from build123d import *

# Parameters (mm, degrees)
PAD_DEPTH = 2.3


with BuildPart() as pad:
    # Sketch001 → Pad (new body, symmetric)
    with BuildSketch(Plane.YZ):
        with BuildLine():
            Line((5, 0), (5, 12))
            Line((5, 12), (8.5, 12))
            Line((8.5, 12), (12.715243, 19.841011))
            ThreePointArc((22.081098, 12.601746), (21.669324, 21.747216), (12.715243, 19.841011))
            Line((8.5, 0), (22.081098, 12.601746))
            Line((5, 0), (8.5, 0))
        make_face()
        with BuildLine():
            Line((-22.081101, 12.60177), (-8.500026, 0))
            Line((-8.500026, 0), (-5.000026, 0))
            Line((-5.000026, 0), (-5.000026, 12))
            Line((-5.000026, 12), (-8.500026, 12))
            Line((-8.500026, 12), (-12.71524, 19.841026))
            ThreePointArc((-12.71524, 19.841026), (-21.66932, 21.747241), (-22.081101, 12.60177))
        make_face()
    extrude(amount=PAD_DEPTH, both=True)


with BuildPart() as obj1:
    # Sketch → Revolution (revolve)
    with BuildSketch(Plane.YZ):
        Polygon((5, 0), (4.19, 0.467654), (4.19, 11.532346), (5, 12), (7.5, 12), (8.5, 0), align=None)
    revolve(axis=Axis((0, 0, 0), (0, 0, 1)))

    # Fusion: union Pad
    add(pad.part)


solid = obj1.part
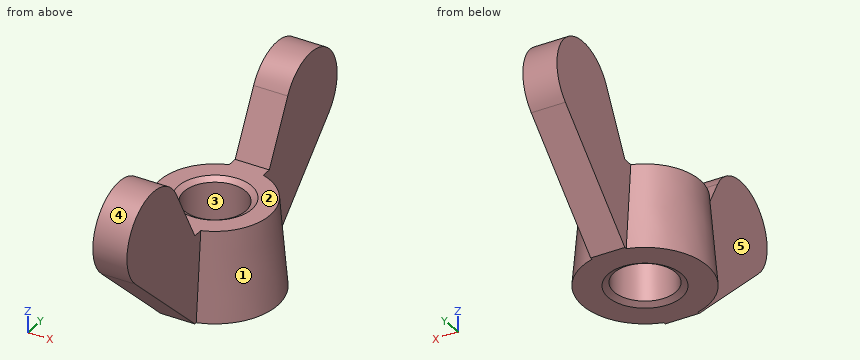
Input: part model. Units: mm. Frame: model coordinates. Face numbers are marked on the shaded views. A direction names the side the tool comes from. Coordinates: 2 decimals unless noted, no trailing zeros. Loops run counter-clockwise (first coordinate to the right, second up) from the corner with the lowest first, then second, coordinate; pieces in that order, holes last. Notation, with made-up numbers: (-8.5, 3.25) - (46.5, 3.25) arc R28 ccw to (46.5, 35.25) - close; hole circle Ø1 at (17, -17.5). An arc over 180 degrees is marked (long way). Answer in a Markdown table with one row per item. Add a question column.
Item 1: Access query for the marked faces 1 and 2. Directions: +Z, -Z, +X, -X, +Y, -Y. A direction counts if a zero-diameter tool reaches every point of the face in a straight line with its end or side. Return the directions, or none.
Item 2: Contact query for flat-ended pins moving along their axis: P1, Ø5, axis at y = -15, z = 10.5, coming from the -X side; P2, Ø5, axis at y = 14.5, z = 15, coming from the +X side; P3, Ø9.5, axis at x = 0, y = 0, coming from the -Z side. Output: stop coordinate, or through.
Item 3: Section query B-B on z = 17.25. Return the cut outline in (x, y).
Item 4: Section query A-A on x = 0. Return the cut outline in (y, z), then the cut area to 3 significant figures.
Item 5: Section query D-D on y = 16. Return the cut outline in (x, z).
Item 6: Section query C-C on z = 10.5. Return the cut outline in (x, y) (3 decimals).
Item 7: Mould query, pull axis X, two halves, no side actions, for the marked faces 3, 4 and 5. Classes: released by +X, released by -X, zero draft, split by the parting line, or undercut.
Item 8: Line query: line 1 along Y through (x, z) = (0, 3.75); line 2 along X through (y, z) = (1, 3); line 3 along X through (y, z) = (11.5, 17.25). Output: solid intervals per line, ascending. Write a range as [from, to].
Recorded:
| question | item | result |
|---|---|---|
| 1 | face 1 | +Z, +X |
| 1 | face 2 | +Z, +X, -X |
| 2 | P1 | x = -2.3 |
| 2 | P2 | x = 2.3 |
| 2 | P3 | z = 0.14 |
| 3 | outline | (-2.3, -23.99) - (2.3, -23.99) - (2.3, -11.32) - (-2.3, -11.32) - close; (-2.3, 11.32) - (2.3, 11.32) - (2.3, 23.99) - (-2.3, 23.99) - close |
| 4 | outline | (-22.08, 12.6) - (-8.5, 0) - (-5, 0) - (-4.19, 0.47) - (-4.19, 11.53) - (-5, 12) - (-8.5, 12) - (-12.72, 19.84) arc R6 ccw (long way) to start; (4.19, 0.47) - (5, 0) - (8.5, 0) - (22.08, 12.6) arc R6 ccw (long way) to (12.72, 19.84) - (8.5, 12) - (5, 12) - (4.19, 11.53) - close |
| 4 | area | 506 mm^2 |
| 5 | outline | (-2.3, 6.96) - (2.3, 6.96) - (2.3, 22.66) - (-2.3, 22.66) - close |
| 6 | outline | (-2.3, -19.816) - (2.3, -19.816) - (2.3, -7.27) arc R7.625 ccw to (2.3, 7.27) - (2.3, 19.816) - (-2.3, 19.816) - (-2.3, 7.27) arc R7.625 ccw to (-2.3, -7.27) - close; hole circle Ø8.38 at (0, 0) |
| 7 | face 3 | undercut |
| 7 | face 4 | zero draft |
| 7 | face 5 | released by -X |
| 8 | line 1 | [-12.54, -4.19], [4.19, 12.54] |
| 8 | line 2 | [-8.19, -4.07], [4.07, 8.19] |
| 8 | line 3 | [-2.3, 2.3] |
